from build123d import *

# Parameters (mm, degrees)
SKETCH1_W           = 21.5
SKETCH1_H           = 38.5
BOSS_EXTRUDE1_DEPTH = 10
SKETCH2_W           = 7.5
SKETCH2_H           = 2
BOSS_EXTRUDE2_DEPTH = 10


with BuildPart() as part:
    # Sketch1 → Boss-Extrude1 (new body)
    with BuildSketch(Plane(origin=(0, 0, 0), x_dir=(1, 0, 0), z_dir=(0, 1, 0))):
        Rectangle(SKETCH1_W, SKETCH1_H)
    extrude(amount=BOSS_EXTRUDE1_DEPTH)

    # Sketch2 → Boss-Extrude2 (add)
    with BuildSketch(Plane.XY.offset(19.25)):
        with Locations((-4.5, 7)):
            Rectangle(SKETCH2_W, SKETCH2_H)
        with Locations((4.5, 4)):
            Rectangle(SKETCH2_W, SKETCH2_H)
        with Locations((-4.5, 4)):
            Rectangle(SKETCH2_W, SKETCH2_H)
        with Locations((4.5, 7)):
            Rectangle(SKETCH2_W, SKETCH2_H)
    extrude(amount=BOSS_EXTRUDE2_DEPTH)


solid = part.part
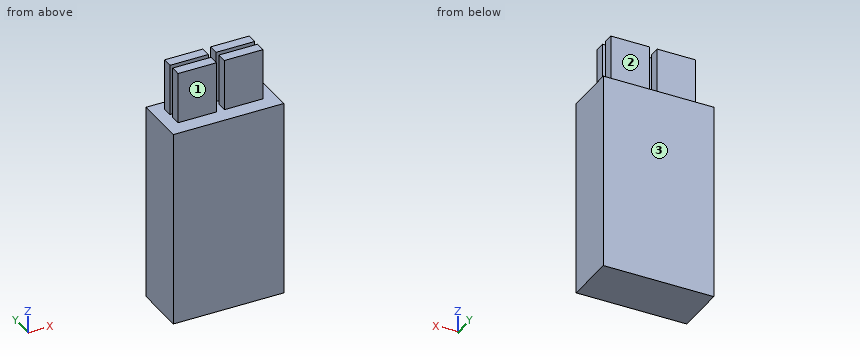
Check sheet for the modelled part. Datum: model origin and axes. Units: mm. Face numbers are marked on the shaded views. A direction names the side the tool comes from. Coordinates: 2 decimals unless noted, no trailing zeros. Write each loop counter-clockwise with the first axis right and the second up, starting at its lowest first coordinate (ties: lowest second). Pieces come first, ordered by that corner, then holes. Notation, with made-up numbers: M 86,-23 L 127,-23 A14 cw 127,-16 Z; hole C 66.25,59 d3. An arc over 180 degrees is marked long. Answer as CSV lines item,"result".
Q1. Material ranges on probe 1 along Y at (x, z) = (-1.5, 26.5); probe 2 along Z at (x, y) = (-3, 9.25), recorded low to high. Write a range as from..to.
Check result:
probe 1,"3..5, 6..8"
probe 2,"-19.25..19.25"
Q2. Set-up check for the marked faces 1, 2 and 3: record each of +Z, -Z, +X, -X, +Y, -Y from which the full face is reachable in a straight line by a thin tool's end or side.
Check result:
face 1,"+Z, +X, -X, -Y"
face 2,"+Z, +X, -X, +Y"
face 3,"+Z, -Z, +X, -X, +Y"
Q3. Cross-section at C-C (y = 1.5). Record the boundary of the cut face in (x, z).
Check result:
outline,"M -10.75,-19.25 L 10.75,-19.25 L 10.75,19.25 L -10.75,19.25 Z"
Q4. Cross-section at A-A (y = 7.5). Record the boundary of the cut face in (x, z), then the cut area to 3 significant figures.
Check result:
outline,"M -10.75,-19.25 L 10.75,-19.25 L 10.75,19.25 L 8.25,19.25 L 8.25,29.25 L 0.75,29.25 L 0.75,19.25 L -0.75,19.25 L -0.75,29.25 L -8.25,29.25 L -8.25,19.25 L -10.75,19.25 Z"
area,"978 mm^2"
Q5. Go/stop test with flat-tipped pins: pin 1 (1 mm diameter, centred on y = 4, z = 22.5, fed in from -X); pin 2 (1.5 mm diameter, centred on x = 3.5, y = 9, fed in from +Z); pin 3 (0.6 mm diameter, centred on y = 7.5, z = 23, fed in from +X). Record where each tip stops, or that it passes through.
Check result:
pin 1,"x = -8.25"
pin 2,"z = 19.25"
pin 3,"x = 8.25"
Q6. Cross-section at B-B (x = -7). Record the boundary of the cut face in (y, z), then the cut area to 3 significant figures.
Check result:
outline,"M 0,-19.25 L 10,-19.25 L 10,19.25 L 8,19.25 L 8,29.25 L 6,29.25 L 6,19.25 L 5,19.25 L 5,29.25 L 3,29.25 L 3,19.25 L 0,19.25 Z"
area,"425 mm^2"
Q7. Cross-section at D-D (x = 8.75). Record the boundary of the cut face in (y, z), then the cut area to 3 significant figures.
Check result:
outline,"M 0,-19.25 L 10,-19.25 L 10,19.25 L 0,19.25 Z"
area,"385 mm^2"
